Autodesk Inventor part; units mm, degrees
ref_plane "YZ Plane" through (0, 0, 0) normal (1, 0, 0) x (0, 1, 0)
ref_plane "XZ Plane" through (0, 0, 0) normal (0, 1, 0) x (-1, 0, 0)
ref_plane "XY Plane" through (0, 0, 0) normal (0, 0, 1) x (1, 0, 0)
sketch "Sketch1" plane through (0, 0, 0) normal (0, 0, 1) x (1, 0, 0)
  circle A0 centre (0, 0) radius 4.699
  dimension "d0" = 9.398
extrude "Extrusion1" add sketch "Sketch1" along normal blind 6.35
sketch "Sketch2" plane through (0, 0, 0) normal (0, 0, -1) x (-1, 0, 0)
  circle A0 centre (0, 0) radius 4.699
  circle A1 centre (0, 0) radius 3.175
  dimension "d3" = 6.35
extrude "Extrusion2" add sketch "Sketch2" along normal blind 12.7 contours A1
thread "Thread1"
sketch "Sketch3" plane through (0, 0, 6.35) normal (0, 0, 1) x (1, 0, 0)
  circle A0 centre (0, 0) radius 4.699
  line L0 (2.7496, 0) -> (1.3748, -2.3813)
  line L1 (1.3748, -2.3813) -> (-1.3748, -2.3813)
  line L2 (-1.3748, -2.3813) -> (-2.7496, 0)
  line L3 (-2.7496, 0) -> (-1.3748, 2.3812)
  line L4 (-1.3748, 2.3812) -> (1.3748, 2.3812)
  line L5 (1.3748, 2.3812) -> (2.7496, 0)
  dimension "d11" = 4.7625
extrude "Extrusion3" cut sketch "Sketch3" against normal blind 5.08 contours L0 L1 L2 L3 L4 L5
properties part number "SHCS bolt"
Design review of the part built by this model. Coordinates are the model's own, in mm. A direction names the side the tool comes from. Round coordinates to 2 decimals unless told otherwise and drop trailing zeros. Write each loop counter-clockwise with the first axis right and the second up, starting at its lowest first coordinate (ties: lowest second). Pieces come first, ordered by that corner, then holes.
Item 1: For faces 1 (the flat face through (2, -2, 6.35)), 2 (the flat face through (-2.072, 1.174, 3.846)), 3 (the cylindrical face through (0.69, 3.1, -6.26)), list the 3-axis set-ups (+Z, -Z, +X, -X, +Y, -Y) from which the entire face can be reached by the end or side of a thin tool; tool diameter is ignored.
Item 2: For probe 1 along Y at (x, z) = (0, 3.75); probe 2 along Z at (x, y) = (3.5, 1.25); probe 3 along Y at (x, z) = (0, -6.5) (3 decimals), list the stretches that pass through material, from the lowest coordinate up.
Item 3: We need section B-B on x = 0. Write out the cut boundary in (y, z) (3 decimals), and give its area (3 significant figures).
Item 4: We need section D-D on y = 3.5. Write out the cut boundary in (x, z).
Item 5: We need section A-A on z = 4.25. Write out the cut boundary in (x, y).
Item 6: Clearance check with flat-ended pins moving along their axes: pin 1 Ø2.5 at (x, y) = (0, 1) entering from +Z; pin 2 Ø5 at (x, z) = (1, -5.5) entering from +Y (3 decimals); pin 3 Ø3 at (y, z) = (-2.5, 2.5) entering from -X; pin 4 Ø0.8 at (x, z) = (0.5, 4.5) entering from +Y. State where each tip first meets the part, or that it passes through.
Item 7: We need section C-C on z = -4.5. Write out the cut boundary in (x, y) (3 decimals), and give its area (3 significant figures).
Item 8: The part is to be moulded in two halves that separate along X. For faces 4 (the flat face through (0, 0, -12.7)), 5 (the cylindrical face through (-0.61, -4.66, 3.13)), 6 (the flat face through (0, -2.381, 4)), say which applies: +X half, -X half, draft (parallel to the pull), parting line (faces both ways), or undercut.
Returned:
1. face 1: +Z, +X, -X, +Y, -Y
1. face 2: +Z
1. face 3: -Z
2. probe 1: y = -4.7 to -2.38, 2.38 to 4.7
2. probe 2: z = 0 to 6.35
2. probe 3: y = -3.175 to 3.175
3. outline: (-4.699, 0) - (-3.175, 0) - (-3.175, -12.7) - (3.175, -12.7) - (3.175, 0) - (4.699, 0) - (4.699, 6.35) - (2.381, 6.35) - (2.381, 1.27) - (-2.381, 1.27) - (-2.381, 6.35) - (-4.699, 6.35) - close
3. area: 116 mm2
4. outline: (-3.14, 0) - (3.14, 0) - (3.14, 6.35) - (-3.14, 6.35) - close
5. outline: circle Ø9.4 at (0, 0); hole (-2.75, 0) - (-1.37, -2.38) - (1.37, -2.38) - (2.75, 0) - (1.37, 2.38) - (-1.37, 2.38) - close
6. pin 1: stops at z = 1.27
6. pin 2: stops at y = 3.175
6. pin 3: stops at x = -4.59
6. pin 4: stops at y = 4.7
7. outline: circle Ø6.35 at (0, 0)
7. area: 31.7 mm2
8. face 4: draft
8. face 5: parting line
8. face 6: undercut
